Could you check a few things on this model? Use its own coordinates, in mm. Round coordinates to 2 decimals unless told otherwise and drop trailing zeros. Loops run counter-clockwise (first coordinate to the right, second up) from the corner with the lowest first, then second, coordinate; pieces in that order, holes last.
from build123d import *

# Parameters (mm, degrees)
F0_R     = 2.45745
F0_R_2   = 4.7625
F1_DEPTH = 3.175


with BuildPart() as f1:
    # F0 (on Front) → F1 (new body)
    with BuildSketch(Plane.XZ):
        with BuildLine():
            Line((-31.75, -12.7), (31.75, -12.7))
            Line((31.75, -12.7), (31.75, 4.7625))
            ThreePointArc((31.75, 4.7625), (29.42516, 10.37516), (23.8125, 12.7))
            Line((23.8125, 12.7), (-23.8125, 12.7))
            ThreePointArc((-23.8125, 12.7), (-29.42516, 10.37516), (-31.75, 4.7625))
            Line((-31.75, 4.7625), (-31.75, -12.7))
        make_face()
        with Locations((-22.225, 0)):
            Circle(F0_R, mode=Mode.SUBTRACT)
        with Locations((-6.35, 0)):
            Circle(F0_R, mode=Mode.SUBTRACT)
        with Locations((15.875, 0)):
            Circle(F0_R_2, mode=Mode.SUBTRACT)
    extrude(amount=F1_DEPTH)


solid = f1.part
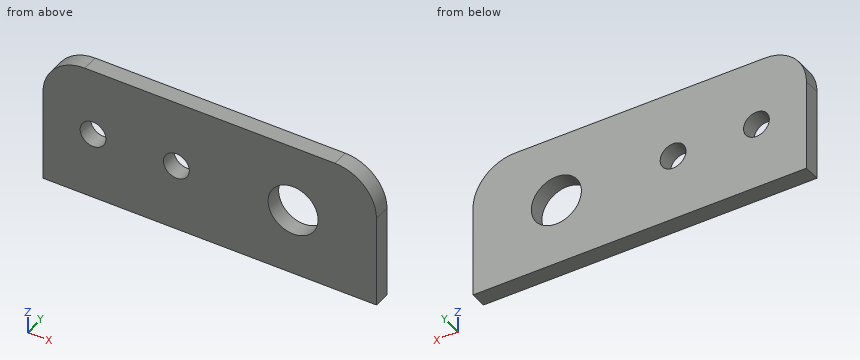
Item 1: Will this pin go through, and if not, where does the flat tip stop? pin 1 (5.5 mm diameter, centred on x = 15.875, z = 0, fed in from -Y).
Results list:
pin 1: passes through
Item 2: If we section it at B-B, the plane z = 0: Count the separate pieces of the cut face and the enclosed holes in it, then the cut area to 3 significant figures.
Results list:
separate pieces: 4
enclosed holes: 0
area: 140 mm2
Item 3: If I drill on line 1 along Z through (x, y) = (-6.35, -1.85); line 2 along X through (y, z) = (-1.4, -3); line 3 along Z through (x, y) = (-20.5, -2.9), over which ranges is the centre line in solid material (lowest first)?
Results list:
line 1: z = -12.7 to -2.46, 2.46 to 12.7
line 2: x = -31.75 to 12.18, 19.57 to 31.75
line 3: z = -12.7 to -1.75, 1.75 to 12.7
Item 4: If we section it at D-D, the plane x = -23: Please give me the cut outline in (y, z) (3 decimals), then the cut area to 3 significant figures.
Results list:
outline: (-3.175, -12.7) - (0, -12.7) - (0, -2.332) - (-3.175, -2.332) - close; (-3.175, 2.332) - (0, 2.332) - (0, 12.7) - (-3.175, 12.7) - close
area: 65.8 mm2
Item 5: If we section it at A-A, the plane x = -6.35: Please give me the cut outline in (y, z) (3 decimals), then the cut area to 3 significant figures.
Results list:
outline: (-3.175, -12.7) - (0, -12.7) - (0, -2.457) - (-3.175, -2.457) - close; (-3.175, 2.457) - (0, 2.457) - (0, 12.7) - (-3.175, 12.7) - close
area: 65.0 mm2
